Design review of the part built by this model. Coordinates are the model's own, in mm. Face numbers are marked on the shaded views. A direction names the side the tool comes from. Coordinates: 2 decimals unless noted, no trailing zeros. Write each loop counter-clockwise with the first axis right and the second up, starting at its lowest first coordinate (ties: lowest second). Pieces come first, ordered by that corner, then holes.
Q1. Add section D-D, the plane z = 10.5. Give the number of separate pieces and of enclosed holes in the cut face, plus the area to 3 significant figures.
Q2. Add section C-C, the plane x = 52.5. Give the boundary of the cut face in (y, z), plus the area to 3 significant figures.
Q3. Add section B-B, the plane y = 14.5. Give the boundary of the cut face in (x, z).
Q4. The part is to be moulded in two halves that separate along X. For the marked faces 1, 2, 3 and 4, say which applies: +X half, -X half, draft (parallel to the pull), parting line (faces both ways), or undercut.
Q5. Add section A-A, the plane x = -16.5. Give the boundary of the cut face in (y, z), plus the area to 3 significant figures.
Q6. Clearance check with a flat-ended pin moving along its axis: pin 1 Ø12.5 at (x, z) = (-5, 15.95) entering from -Y. State where the tip first meets the part, or that it passes through.
Q7. To check wall thickness, follow probe 1 along Z at (x, y) = (17, -12); probe 2 along X at (y, z) = (-14, 19); probe 3 along X at (y, z) = (-12, 19.5). State the ranges of each line that lie inside material, in increasing order.
Q8. Machinability: for the marked faces 5, 6 and 7, which of the approach directions +Z, -Z, +X, -X, +Y, -Y give a long, thin tool a straight path to every point of the face, cutting with its end or side? Answer none if there is none.
from build123d import *

# Parameters (mm, degrees)
F0_W           = 9.5
F0_H           = 6
F0_W_2         = 67
F0_H_2         = 46
F0_W_3         = 43.5
F1_DEPTH       = 31.9024
F2_D           = 6.5
F5_D           = 13.716
F5_DEPTH       = 16.5
F5_TIP         = 4.1207021253
F5_ON_F4_D     = 13.716
F5_ON_F4_DEPTH = 16.5
F5_ON_F4_TIP   = 4.1207021253


with BuildPart() as f1:
    # F0 (on Top) → F1 (new body)
    with BuildSketch(Plane.XY):
        with Locations((55.25, -23)):
            Rectangle(F0_W, F0_H)
        with Locations((17, -23)):
            Rectangle(F0_W_2, F0_H)
        with Locations((55.25, 3)):
            Rectangle(F0_W, F0_H_2)
        with Locations((-38.25, -23)):
            Rectangle(F0_W_3, F0_H)
        with Locations((17, 3)):
            Rectangle(F0_W_2, F0_H_2)
        with Locations((-38.25, 3)):
            Rectangle(F0_W_3, F0_H_2)
    extrude(amount=F1_DEPTH)

    # F2 (through all)
    with Locations(Plane(origin=(0, 0, 0), x_dir=(1, 0, 0), z_dir=(0, 0, -1))):
        with Locations((-16.5, 20), (50.5, 20)):
            Hole(F2_D / 2)

    # F5
    with Locations(Plane.XZ.offset(26)):
        with Locations((-5, 15.9512), (17, 15.9512), (39, 15.9512)):
            Hole(F5_D / 2, depth=F5_DEPTH)
            with Locations((0, 0, -(F5_DEPTH + F5_TIP / 2))):  # 118° drill point
                Cone(0, F5_D / 2, F5_TIP, mode=Mode.SUBTRACT)

    # F5 on F4
    with Locations(Plane(origin=(0, 26, 0), x_dir=(-1, 0, 0), z_dir=(0, 1, 0))):
        with Locations((-28, 15.9512), (-6, 15.9512)):
            Hole(F5_ON_F4_D / 2, depth=F5_ON_F4_DEPTH)
            with Locations((0, 0, -(F5_ON_F4_DEPTH + F5_ON_F4_TIP / 2))):  # 118° drill point
                Cone(0, F5_ON_F4_D / 2, F5_ON_F4_TIP, mode=Mode.SUBTRACT)


solid = f1.part
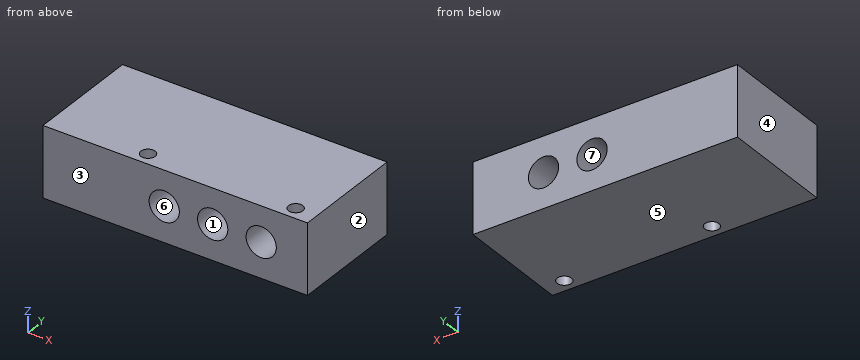
Here are the results:
1. separate pieces: 1
1. enclosed holes: 2
1. area: 5,460 mm2
2. outline: (-26, 0) - (-22.56, 0) - (-22.56, 31.9) - (-26, 31.9) - close; (-17.44, 0) - (26, 0) - (26, 31.9) - (-17.44, 31.9) - close
2. area: 1,500 mm2
3. outline: (-60, 0) - (60, 0) - (60, 31.9) - (-60, 31.9) - close; hole circle Ø13.72 at (6, 15.95); hole circle Ø13.72 at (28, 15.95)
4. face 1: undercut
4. face 2: +X half
4. face 3: draft
4. face 4: -X half
5. outline: (-26, 0) - (-23.25, 0) - (-23.25, 31.9) - (-26, 31.9) - close; (-16.75, 0) - (26, 0) - (26, 31.9) - (-16.75, 31.9) - close
5. area: 1,450 mm2
6. pin 1: stops at y = -9.14
7. probe 1: z = 0 to 9.09, 22.81 to 31.9
7. probe 2: x = -60 to -11.14, 1.14 to 10.86, 23.14 to 32.86, 45.14 to 60
7. probe 3: x = -60 to -10.87, 0.87 to 11.13, 22.87 to 33.13, 44.87 to 60
8. face 5: -Z, +X, -X, +Y, -Y
8. face 6: -Y
8. face 7: +Y
